Check sheet for the modelled part. Datum: model origin and axes. Units: mm. Face numbers are marked on the shaded views. A direction names the side the tool comes from. Give positions to 0.01 mm unless a question says otherwise; leave off trailing zeros. Write each loop counter-clockwise with the first axis right and the second up, starting at its lowest first coordinate (ties: lowest second). Pieces come first, ordered by that corner, then holes. Notation, with made-up numbers: (36, 82) -> (47, 82) arc R25 cw to (47, 95) -> close; hole circle Ø11 at (82, 69). An arc over 180 degrees is marked (long way). Use a Markdown table: item, result. Add a question column.
1. Scan lines: probe 1 along Z at (x, y) = (-57.5, 32); probe 2 along Z at (x, y) = (29.5, -68); probe 3 along X at (y, z) = (0, 166). Record each from-to range of solid material in increasing order. Write a range as [from, to].
2. Release check for a two-part mould opening along Z. For the marked faces 1, 2 and 3 record: released by +Z, released by -Z, zero draft, split by the parting line, or undercut.
3. Cross-section at B-B (x = -21). Enter the section's corners in (y, z).
4. Gauge pin test, flat ends, axial feed: P1, Ø1, axis at x = 16, z = 330, coming from the +Y side; P2, Ø10, axis at x = -22.5, z = 86, coming from the +Y side; P3, Ø11, axis at x = 41.5, y = 79.77, coming from the -Z side; P4, Ø20.5, axis at x = 0, y = 0, coming from the +Z side. Record the tip position at first contact, or that the pin passes through.
5. Cross-section at A-A (z = 75.5). Enter the section's corners in (x, y), then the cut area to 3 significant figures.
6. Cross-section at C-C (y = 124). Enter the section's corners in (x, z) (3 decimals), then the cut area to 3 significant figures.
7. Set-up check for the marked faces 4, 5 and 6: record each of +Z, -Z, +X, -X, +Y, -Y from which the full face is reachable in a straight line by a thin tool's end or side.
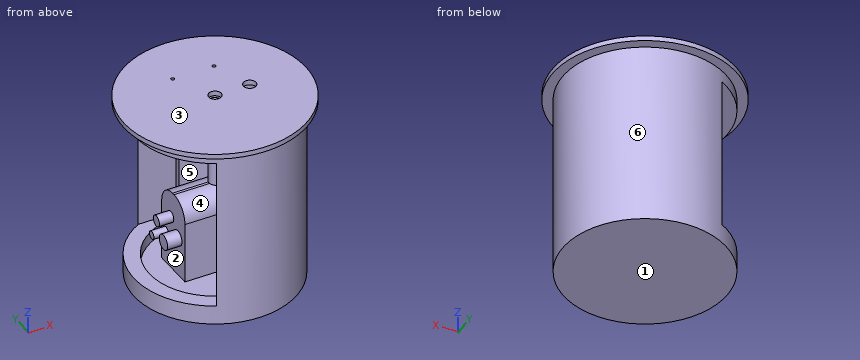
from build123d import *

# Parameters (mm, degrees)
CROQUIS1_R              = 162.5
SALIENTE_EXTRUIR1_DEPTH = 370
CROQUIS2_R              = 132
CORTAR_EXTRUIR1_DEPTH   = 417
CROQUIS3_W              = 307.465117838
CROQUIS3_H              = 287.064574964
CORTAR_EXTRUIR2_DEPTH   = 417
CROQUIS4_R              = 182.5
CROQUIS4_R_2            = 12.7
CROQUIS4_R_3            = 3.5
SALIENTE_EXTRUIR2_DEPTH = 10
SALIENTE_EXTRUIR3_DEPTH = 84
CROQUIS6_R              = 11.039446922
CROQUIS6_R_2            = 15.273211948
CROQUIS6_R_3            = 8.18574154
SALIENTE_EXTRUIR4_DEPTH = 113
CROQUIS7_R              = 12.7
SALIENTE_EXTRUIR5_DEPTH = 351


with BuildPart() as part:
    # Croquis1 → Saliente-Extruir1 (new body)
    with BuildSketch(Plane.XY):
        Circle(CROQUIS1_R)
    extrude(amount=SALIENTE_EXTRUIR1_DEPTH)

    # Croquis2 → Cortar-Extruir1 (cut)
    with BuildSketch(Plane.XY.offset(15)):
        Circle(CROQUIS2_R)
    extrude(amount=CORTAR_EXTRUIR1_DEPTH, mode=Mode.SUBTRACT)

    # Croquis3 → Cortar-Extruir2 (cut)
    with BuildSketch(Plane(origin=(0, 0, 0), x_dir=(0, 0, -1), z_dir=(1, 0, 0))):
        with Locations((-192.5, 0)):
            Rectangle(CROQUIS3_W, CROQUIS3_H)
    extrude(amount=-CORTAR_EXTRUIR2_DEPTH, mode=Mode.SUBTRACT)

    # Croquis4 → Saliente-Extruir2 (add)
    with BuildSketch(Plane.XY.offset(370)):
        Circle(CROQUIS4_R)
        Circle(CROQUIS4_R_2, mode=Mode.SUBTRACT)
        with Locations((70, 0)):
            Circle(CROQUIS4_R_2, mode=Mode.SUBTRACT)
        with Locations((-41.5, 79.772762666)):
            Circle(CROQUIS4_R_3, mode=Mode.SUBTRACT)
        with Locations((41.5, 79.772762666)):
            Circle(CROQUIS4_R_3, mode=Mode.SUBTRACT)
    extrude(amount=SALIENTE_EXTRUIR2_DEPTH)



with BuildPart() as body_2:
    # Croquis5 → Saliente-Extruir3 (new body)
    with BuildSketch(Plane(origin=(0, 0, 0), x_dir=(0, 0, -1), z_dir=(1, 0, 0))):
        with BuildLine():
            Line((-155.328170247, 42.685027874), (-31.585382794, 42.685027874))
            Line((-31.585382794, 42.685027874), (-31.585382794, -42.685027874))
            Line((-31.585382794, -42.685027874), (-155.328170247, -42.685027874))
            ThreePointArc((-155.328170247, -42.685027874), (-183.612441494, -30.969299122), (-195.328170247, -2.685027874))
            Line((-195.328170247, -2.685027874), (-195.328170247, 2.685027874))
            ThreePointArc((-195.328170247, 2.685027874), (-183.612441494, 30.969299122), (-155.328170247, 42.685027874))
        make_face()
    extrude(amount=-SALIENTE_EXTRUIR3_DEPTH)

    # Croquis6 → Saliente-Extruir4 (add)
    with BuildSketch(Plane(origin=(0, 0, 0), x_dir=(0, 0, -1), z_dir=(1, 0, 0))):
        with Locations((-140.988957086, 9.44161276)):
            Circle(CROQUIS6_R)
        with Locations((-110.953177837, -16.572410972)):
            Circle(CROQUIS6_R_2)
        with Locations((-99.615024167, 26.769678135)):
            Circle(CROQUIS6_R_3)
    extrude(amount=-SALIENTE_EXTRUIR4_DEPTH)


with BuildPart() as part_1:
    add(part.part)

    add(body_2.part)  # Saliente-Extruir5 merges body 2
    # Croquis7 → Saliente-Extruir5 (add)
    with BuildSketch(Plane.XY.offset(15)):
        Circle(CROQUIS7_R)
    extrude(amount=SALIENTE_EXTRUIR5_DEPTH)


solid = part_1.part
Worked answers:
| question | item | result |
|---|---|---|
| 1 | probe 1 | z = [0, 15], [31.59, 182.54], [370, 380] |
| 1 | probe 2 | z = [0, 15], [370, 380] |
| 1 | probe 3 | x = [-84, 12.7], [132, 162.5] |
| 2 | face 1 | released by -Z |
| 2 | face 2 | undercut |
| 2 | face 3 | released by +Z |
| 3 | outline | (-181.29, 370) -> (-161.14, 370) -> (-161.14, 0) -> (161.14, 0) -> (161.14, 370) -> (181.29, 370) -> (181.29, 380) -> (-181.29, 380) -> close; (-42.69, 31.59) -> (42.69, 31.59) -> (42.69, 155.33) arc R40 ccw to (2.69, 195.33) -> (-2.69, 195.33) arc R40 ccw to (-42.69, 155.33) -> close; hole (-143.53, 38.77) -> (-130.32, 38.77) -> (-130.32, 15) -> (130.32, 15) -> (130.32, 38.77) -> (143.53, 38.77) -> (143.53, 346.23) -> (130.32, 346.23) -> (130.32, 370) -> (-130.32, 370) -> (-130.32, 346.23) -> (-143.53, 346.23) -> close |
| 4 | P1 | stops at y = 161.76 |
| 4 | P2 | stops at y = 161.55 |
| 4 | P3 | stops at z = 0 |
| 4 | P4 | stops at z = 366 |
| 5 | outline | (-84, -42.69) -> (0, -42.69) -> (0, -12.7) arc R12.7 ccw to (0, 12.7) -> (0, 42.69) -> (-84, 42.69) -> close; (-76.19, -143.53) arc R162.5 ccw (long way) to (-76.19, 143.53) -> (0, 143.53) -> (0, 132) arc R132 cw to (0, -132) -> (0, -143.53) -> close |
| 5 | area | 23,500 mm² |
| 6 | outline | (-133.904, 370) -> (-105.025, 370) -> (-105.025, 346.233) -> (-45.255, 346.233) -> (-45.255, 370) -> (45.255, 370) -> (45.255, 15) -> (-45.255, 15) -> (-45.255, 38.767) -> (-105.025, 38.767) -> (-105.025, 0) -> (105.025, 0) -> (105.025, 370) -> (133.904, 370) -> (133.904, 380) -> (-133.904, 380) -> close |
| 6 | area | 29,900 mm² |
| 7 | face 4 | -X |
| 7 | face 5 | none |
| 7 | face 6 | -Z |
